from build123d import *

# Parameters (mm, degrees)
ESTRUSIONE_ESTRUSIONE1_DEPTH = 2


with BuildPart() as part:
    # Schizzo1 → Estrusione-Estrusione1 (new body)
    with BuildSketch(Plane.XY):
        with BuildLine():
            Line((-1.707609412, 24.419952295), (-1.716801654, 24.55140748))
            ThreePointArc((-1.716801654, 24.55140748), (-1.652997524, 25.409995743), (-1.347968624, 26.215105762))
            Line((-1.347968624, 26.215105762), (-0.639867053, 27.492554813))
            ThreePointArc((-0.639867053, 27.492554813), (0, -27.5), (0.639867053, 27.492554813))
            Line((0.639867053, 27.492554813), (1.347968624, 26.215105762))
            ThreePointArc((1.347968624, 26.215105762), (1.652997524, 25.409995743), (1.716801654, 24.55140748))
            Line((1.716801654, 24.55140748), (1.707609412, 24.419952295))
            ThreePointArc((1.707609412, 24.419952295), (1.937229379, 23.709678932), (2.594758219, 23.356310278))
            ThreePointArc((2.594758219, 23.356310278), (0, -23.5), (-2.594758219, 23.356310278))
            ThreePointArc((-2.594758219, 23.356310278), (-1.937229379, 23.709678932), (-1.707609412, 24.419952295))
        make_face()
    extrude(amount=ESTRUSIONE_ESTRUSIONE1_DEPTH)


solid = part.part
Geometry check sheet. Reference: the model listing, model coordinates, mm. A direction names the side the tool comes from. Round coordinates to 2 decimals unless told otherwise and drop trailing zeros. Loops run counter-clockwise (first coordinate to the right, second up) from the corner with the lowest first, then second, coordinate; pieces in that order, holes last.
Item 1: Access from +Z, -Z, +X, -X, +Y, -Y to the whole of each face (thin tool, end or side, straight path). Record for faces 4 (the flat face through (0.99, 26.86, 0.99)), 5 (the flat face through (8, -22.3, 2)).
Item 2: Mould release check, pull along X, two halves, no side actions. Record for faces 1 (the cylindrical face through (1, -23.48, 0.99)), 2 (the flat face through (8, -22.3, 0)), 3 (the cylindrical face through (-1.2, -27.474, 0.986)): pulls with the +X half, pulls with the -X half, needs draft (parallel to the pull), parting line crosses it, or undercut.
Item 3: Cross-section at B-B on x = 16. Record the boundary of the cut face in (y, z).
Item 4: Thickness scan on line 1 (X direction, y = 0, z = 0.95); line 2 (Y direction, x = 0, z = 1.4); line 3 (X direction, y = -7, z = 1.35). Record the ranges inside material, lowest first.
Item 5: Cross-section at A-A on y = 0. Record the boundary of the cut face in (x, z), then the cut area to 3 significant figures.
Item 6: Gauge pin test, flat end, axial feed: pin 1 (1 mm diameter, centred on y = -10.5, z = 1, fed in from -X). Record the tip position at first contact, or that the pin passes through.
Item 7: Cross-section at D-D on x = 0. Record the boundary of the cut face in (y, z), then the cut area to 3 significant figures.
Item 8: Cross-section at C-C on z = 0.9. Record the boundary of the cut face in (x, y).
Answer sheet:
1. face 4: +Z, -Z
1. face 5: +Z, +X, -X, +Y, -Y
2. face 1: undercut
2. face 2: needs draft
2. face 3: parting line crosses it
3. outline: (-22.37, 0) - (-17.21, 0) - (-17.21, 2) - (-22.37, 2) - close; (17.21, 0) - (22.37, 0) - (22.37, 2) - (17.21, 2) - close
4. line 1: x = -27.5 to -23.5, 23.5 to 27.5
4. line 2: y = -27.5 to -23.5
4. line 3: x = -26.59 to -22.43, 22.43 to 26.59
5. outline: (-27.5, 0) - (-23.5, 0) - (-23.5, 2) - (-27.5, 2) - close; (23.5, 0) - (27.5, 0) - (27.5, 2) - (23.5, 2) - close
5. area: 16.0 mm2
6. pin 1: stops at x = -25.62
7. outline: (-27.5, 0) - (-23.5, 0) - (-23.5, 2) - (-27.5, 2) - close
7. area: 8.00 mm2
8. outline: (-2.59, 23.36) arc R1 ccw to (-1.71, 24.42) - (-1.72, 24.55) arc R3 cw to (-1.35, 26.22) - (-0.64, 27.49) arc R27.5 ccw (long way) to (0.64, 27.49) - (1.35, 26.22) arc R3 cw to (1.72, 24.55) - (1.71, 24.42) arc R1 ccw to (2.59, 23.36) arc R23.5 cw (long way) to start
